Design review of the part built by this model. Coordinates are the model's own, in mm. A direction names the side the tool comes from. Coordinates: 2 decimals unless noted, no trailing zeros. Loops run counter-clockwise (first coordinate to the right, second up) from the corner with the lowest first, then second, coordinate; pieces in that order, holes last.
Q1. Machinability: for faces 5 (the face through (493, 0, 493)), 6 (the face through (218, 40, 276)), which of the approach directions +Z, -Z, +X, -X, +Y, -Y give a long, thin tool a straight path to every point of the face, cutting with its end or side? Answer none if there is none.
Q2. Add section A-A on x = 276.5. Give the boundary of the cut face in (y, z).
Q3. Add section C-C on y = 49. Give the boundary of the cut face in (x, z), and give its area (3 significant figures).
Q4. For P1, Ø5, axis at x = 533, y = 26, coming from the +Z side; P2, Ø10, axis at y = 9.5, z = 597, coming from the +X side, all flat-tipped, find the tip position at first contact; note any pin that passes through.
Q5. Add section D-D on z = 709. Give the boundary of the cut face in (x, y).
Q6. Wall thickness on probe 1 along X at (y, z) = (22, 276); probe 2 along X at (y, z) = (53, 284); probe 3 along Z at (x, y) = (462, 51.5): over which ranges is each line inside the solid? List them lowest first.
Q7. Add section B-B on z = 276.5. Give the boundary of the cut face in (x, y), and give its area (3 significant figures).
Q8. Draft analysis for pull direction Z (two halves, no side actions). For faces 1 (the face through (222, 30, 1000)), 2 (the face through (493, 30, 0)), 3 (the face through (1000, 30, 222)), 4 (the face through (219.88, 20.28, 263.93)), state which applies: released by +Z, released by -Z, zero draft, split by the parting line, or undercut.
```python
from build123d import *

# Parameters (mm, degrees)
SKIZZE1_W                       = 1000
SKIZZE1_H                       = 60
AUFSATZ_LINEAR_AUSTRAGEN1_DEPTH = 1000
SCHNITT_LINEAR_AUSTRAGEN1_DEPTH = 1000
SKIZZE3_R                       = 58
SCHNITT_LINEAR_AUSTRAGEN2_DEPTH = 61
SKIZZE4_W                       = 120
SKIZZE4_H                       = 120
SCHNITT_LINEAR_AUSTRAGEN3_DEPTH = 20


with BuildPart() as part:
    # Skizze1 → Aufsatz-Linear austragen1 (new body)
    with BuildSketch(Plane.XY):
        with Locations((500, 30)):
            Rectangle(SKIZZE1_W, SKIZZE1_H)
    extrude(amount=AUFSATZ_LINEAR_AUSTRAGEN1_DEPTH)

    # Skizze2 → Schnitt-Linear austragen1 (cut)
    with BuildSketch(Plane(origin=(0, 60, 0), x_dir=(1, 0, 0), z_dir=(0, 1, 0))):
        with BuildLine():
            Line((1000, -1000), (1000, -450))
            ThreePointArc((1000, -450), (838.908729653, -838.908729653), (450, -1000))
            Line((450, -1000), (1000, -1000))
        make_face()
    extrude(amount=-SCHNITT_LINEAR_AUSTRAGEN1_DEPTH, mode=Mode.SUBTRACT)

    # Skizze3 → Schnitt-Linear austragen2 (cut, through all)
    with BuildSketch(Plane(origin=(0, 60, 0), x_dir=(1, 0, 0), z_dir=(0, 1, 0))):
        with Locations(Location((276.5, -276.5, 0), (0, 0, 270))):  # turned: the seam where the file's is
            Circle(SKIZZE3_R)
    extrude(amount=-SCHNITT_LINEAR_AUSTRAGEN2_DEPTH, mode=Mode.SUBTRACT)

    # Skizze4 → Schnitt-Linear austragen3 (cut)
    with BuildSketch(Plane(origin=(0, 60, 0), x_dir=(1, 0, 0), z_dir=(0, 1, 0))):
        with Locations((276.5, -276.5)):
            Rectangle(SKIZZE4_W, SKIZZE4_H)
    extrude(amount=-SCHNITT_LINEAR_AUSTRAGEN3_DEPTH, mode=Mode.SUBTRACT)


solid = part.part
```
Entries:
1. face 5: +Z, -Z, +X, -X, -Y
1. face 6: +Y
2. outline: (0, 0) - (60, 0) - (60, 216.5) - (40, 216.5) - (40, 218.5) - (0, 218.5) - close; (0, 334.5) - (40, 334.5) - (40, 336.5) - (60, 336.5) - (60, 1000) - (0, 1000) - close
3. outline: (0, 0) - (1000, 0) - (1000, 450) arc R550 ccw to (450, 1000) - (0, 1000) - close; hole (216.5, 216.5) - (336.5, 216.5) - (336.5, 336.5) - (216.5, 336.5) - close
3. area: 921,000 mm2
4. P1: stops at z = 994.08
4. P2: stops at x = 981.35
5. outline: (0, 0) - (935.2, 0) - (935.2, 60) - (0, 60) - close
6. probe 1: x = 0 to 218.5, 334.5 to 1000
6. probe 2: x = 0 to 216.5, 336.5 to 1000
6. probe 3: z = 0 to 999.87
7. outline: (0, 0) - (218.5, 0) - (218.5, 40) - (216.5, 40) - (216.5, 60) - (0, 60) - close; (334.5, 0) - (1000, 0) - (1000, 60) - (336.5, 60) - (336.5, 40) - (334.5, 40) - close
7. area: 53,000 mm2
8. face 1: released by +Z
8. face 2: released by -Z
8. face 3: zero draft
8. face 4: undercut
